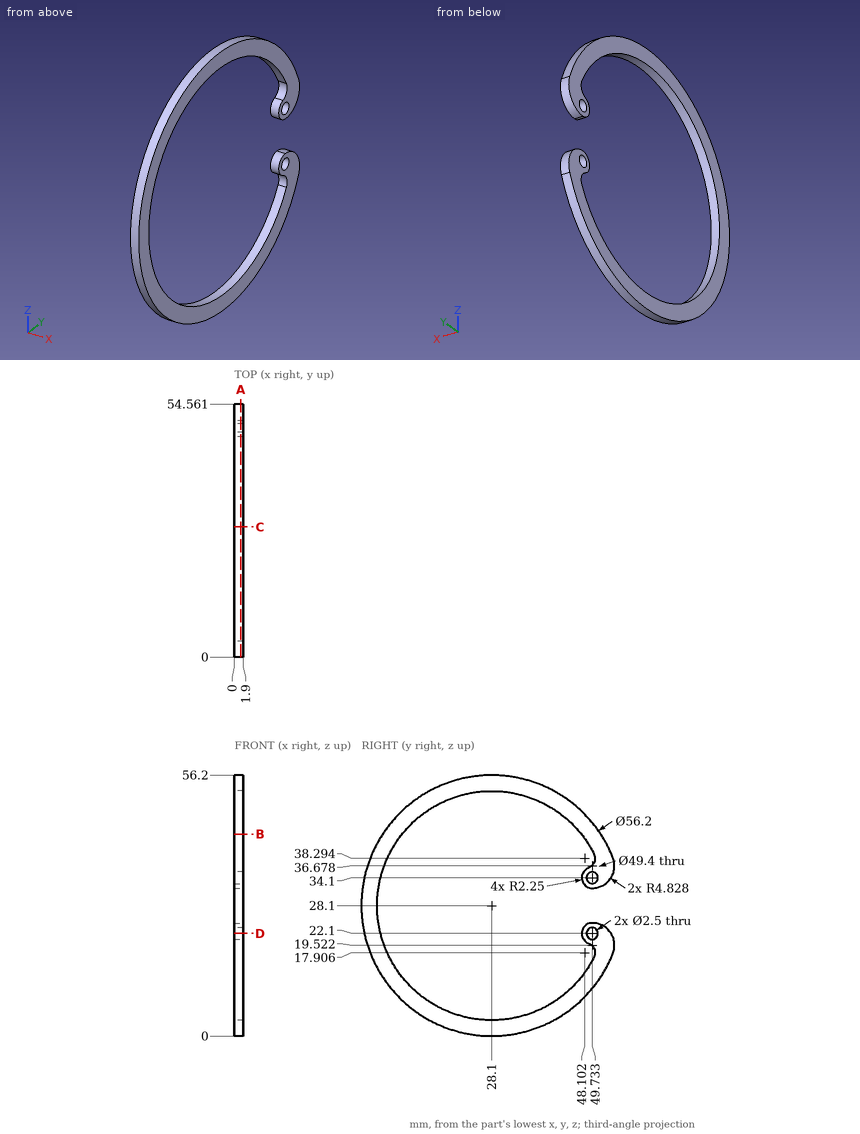
Input: dimensioned drawing with shaded views. Units: mm. Origin: part minimum x, y, z. Coordinates: 2 decimals unless noted, no trailing zeros. Write each loop counter-clockwise with the first axis right and the second up, starting at its lowest first coordinate (ties: lowest second). Pieces come first, ordered by that corner, then holes. Notation, with made-up numbers: M -14,32 L 6,32 A10 cw 6,45 Z; hole C -4,-25.5 d2. An arc over 180 degrees is marked long. Answer as a JSON object with one key per item and string values. Group by question number.
(1) Section D-D on z = 22.1. Output: boundary loops of the cut face in (x, y) (1 decimal).
(2) Section C-C on y = 28.1. Output: boundary loops of the cut face in (x, z), plus the area to 3 significant figures.
(3) Ray query, line 1 along Z through (x, y) = (1, 28.1); line 2 along Y through (x, z) = (0.9, 22.1) (1 decimal); line 3 along Z through (x, y) = (0.6, 34.5). Return the intervals inside material, ascending. Write a range as [from, to].
(4) Section B-B on z = 43.5. Output: boundary loops of the cut face in (x, y) (1 decimal).
(5) Contact query for flat-ended pins moving along their axis: P1, Ø4, axis at y = 49.73, z = 34.1, coming from the -X side; P2, Ø2, axis at y = 49.73, z = 22.1, coming from the +X side. Output: stop coordinate, or through.
(6) Section A-A on x = 1.4. Give the number of separate pieces and of enclosed holes in the cut face, plus the area to 3 significant figures.
Result set:
{
 "1": {"outline": "M 0,0.6 L 1.9,0.6 L 1.9,4.1 L 0,4.1 Z; M 0,47.5 L 1.9,47.5 L 1.9,48.5 L 0,48.5 Z; M 0,51 L 1.9,51 L 1.9,53.8 L 0,53.8 Z"},
 "2": {"outline": "M 0,0 L 1.9,0 L 1.9,3.4 L 0,3.4 Z; M 0,52.8 L 1.9,52.8 L 1.9,56.2 L 0,56.2 Z", "area": "12.9 mm2"},
 "3": {"line 1": "z = [0, 3.4], [52.8, 56.2]", "line 2": "y = [0.6, 4.1], [47.5, 48.5], [51, 53.8]", "line 3": "z = [0.74, 4.24], [51.96, 55.46]"},
 "4": {"outline": "M 0,4.6 L 1.9,4.6 L 1.9,8.8 L 0,8.8 Z; M 0,47.4 L 1.9,47.4 L 1.9,51.6 L 0,51.6 Z"},
 "5": {"P1": "stops at x = 0", "P2": "passes through"},
 "6": {"separate pieces": "1", "enclosed holes": "2", "area": "550 mm2"}
}
